For this review, take the finished solid that the model builds, in its own axes (mm). A direction names the side the tool comes from. Give positions to 0.01 mm unless a question says otherwise; leave off trailing zeros. Order: outer loops, then holes, each group sorted by start corner. A loop starts at its lowest first (then second) coordinate and runs counter-clockwise, first axis right, second up. Notation, with made-up numbers: (-34, 6) - (-11, 6) arc R23 cw to (-11, 44) - close; hole circle Ø5 at (-1, 75.25). An arc over 180 degrees is marked (long way). Use a Markdown table: item, result. Add a question column.
1) We need section B-B on z = 10. Write out the cut boundary in (x, y).
2) Machinability: for faces 4 (the face through (19, -29, 5)), 5 (the face through (20, -53, 2)), which of the approach directions +Z, -Z, +X, -X, +Y, -Y give a long, thin tool a straight path to every point of the face, cutting with its end or side? Answer none if there is none.
3) We need section A-A on x = 19.5. Write out the cut boundary in (y, z).
4) Wall thickness on L1, parallel to Z at x = 35, y = -2.5; L2, parallel to X at y = -1.5, z = 41; L3, parallel to Z at x = 19.5, y = -3.9: over which ranges is each line inside the solid? List them lowest first.
5) We need section C-C on x = 4. Write out the cut boundary in (y, z).
6) We need section D-D on y = -13. Write out the cut boundary in (x, z).
7) Mouldability with a two-part tool opening along Z and no side actions: class faces 1 (the face through (29.259, -2.465, 19.924)), 2 (the face through (0, -17, 4)), 3 (the face through (19, -2, 45)) as released by +Z, released by -Z, zero draft, split by the parting line, or undercut.
8) Clearance check with flat-ended pins moving along their axes: P1, Ø8, axis at x = 28.5, y = -10, coming from the +Z side; P2, Ø5, axis at x = 12.5, z = 9.5, coming from the -Y side; P3, Ø1, axis at x = 8, y = -16, coming from the -Z side; P4, Ø1.8, axis at x = 4, z = 10, coming from the -Y side. State where each tip first meets the part, or that it passes through.
Autodesk Inventor part; units mm, degrees
ref_plane "YZ Plane" through (0, 0, 0) normal (1, 0, 0) x (0, 1, 0)
ref_plane "XZ Plane" through (0, 0, 0) normal (0, 1, 0) x (-1, 0, 0)
ref_plane "XY Plane" through (0, 0, 0) normal (0, 0, 1) x (1, 0, 0)
sketch "Sketch1" plane through (0, 0, 0) normal (0, 0, 1) x (1, 0, 0)
  line L0 (0, 0) -> (39, 0)
  line L1 (39, 0) -> (39, -53)
  line L2 (39, -53) -> (0, -53)
  line L3 (0, -53) -> (0, 0)
  dimension "d0" = 39
  dimension "d1" = 53
extrude "Extrusion1" add sketch "Sketch1" along normal blind 5
sketch "Sketch2" plane through (0, 0, 5) normal (0, 0, 1) x (1, 0, 0)
  line L0 (39, 0) -> (0, 0)
  line L1 (39, -53) -> (39, 0)
  line L2 (0, 0) -> (39, 0)
  line L3 (39, 0) -> (39, -5)
  line L4 (39, -5) -> (0, -5)
  line L5 (0, -5) -> (0, 0)
  dimension "d4" = 5
extrude "Extrusion2" add sketch "Sketch2" along normal blind 40
sketch "Sketch3" plane through (0, -5, 5) normal (0, -1, 0) x (1, 0, 0)
  line L0 (0, 0) -> (0, 40)
  line L1 (0, 0) -> (39, 0)
  point P0 (0, -5)
  point P1 (19.5, 20)
  point P2 (4, 5)
  point P3 (4, 36)
  point P4 (35, 5)
  point P5 (35, 36)
  dimension "d7" = 19.5
  dimension "d8" = 20
  dimension "d9" = 5
  dimension "d10" = 4
  dimension "d13" = 31
  dimension "d16" = 31
hole "Hole1" at (19.5, -5, 25) direction (0, 1, 0) diameter 22 end through all
hole "Hole2" at (4, -5, 10) at (4, -5, 41) at (35, -5, 41) at (35, -5, 10) direction (0, 1, 0) diameter 3 end through all
properties part number "head-baseblate" material "Aluminum 6061"
Checked values:
| question | item | result |
|---|---|---|
| 1 | outline | (0, -5) - (2.5, -5) - (2.5, 0) - (0, 0) - close; (5.5, -5) - (33.5, -5) - (33.5, 0) - (5.5, 0) - close; (36.5, -5) - (39, -5) - (39, 0) - (36.5, 0) - close |
| 2 | face 4 | +Z, +X, -X, -Y |
| 2 | face 5 | +Z, -Z, +X, -X, -Y |
| 3 | outline | (-53, 0) - (0, 0) - (0, 14) - (-5, 14) - (-5, 5) - (-53, 5) - close; (-5, 36) - (0, 36) - (0, 45) - (-5, 45) - close |
| 4 | L1 | 0 to 8.5, 11.5 to 39.5, 42.5 to 45 |
| 4 | L2 | 0 to 2.5, 5.5 to 33.5, 36.5 to 39 |
| 4 | L3 | 0 to 14, 36 to 45 |
| 5 | outline | (-53, 0) - (0, 0) - (0, 8.5) - (-5, 8.5) - (-5, 5) - (-53, 5) - close; (-5, 11.5) - (0, 11.5) - (0, 39.5) - (-5, 39.5) - close; (-5, 42.5) - (0, 42.5) - (0, 45) - (-5, 45) - close |
| 6 | outline | (0, 0) - (39, 0) - (39, 5) - (0, 5) - close |
| 7 | face 1 | undercut |
| 7 | face 2 | zero draft |
| 7 | face 3 | released by +Z |
| 8 | P1 | z = 5 |
| 8 | P2 | y = -5 |
| 8 | P3 | z = 0 |
| 8 | P4 | through |
